from build123d import *

# Parameters (mm, degrees)
SKETCH1_R           = 11
SKETCH1_R_2         = 6.5
BOSS_EXTRUDE1_DEPTH = 2.75
SKETCH1_3_R         = 12.5
SKETCH1_3_R_2       = 11
SKETCH1_3_R_3       = 6.5
SKETCH1_3_R_4       = 5
BOSS_EXTRUDE2_DEPTH = 3
CHAMFER1_SIZE       = 0.3


with BuildPart() as part:
    # Sketch1 → Boss-Extrude1 (new, symmetric)
    with BuildSketch(Plane(origin=(0, 0, 0), x_dir=(1, 0, 0), z_dir=(0, 1, 0))):
        with Locations(Location((0, 0, 0), (0, 0, 270))):
            Circle(SKETCH1_R)
        with Locations(Location((0, 0, 0), (0, 0, 270))):
            Circle(SKETCH1_R_2, mode=Mode.SUBTRACT)
    extrude(amount=BOSS_EXTRUDE1_DEPTH, both=True)

    # Sketch1_3 → Boss-Extrude2 (add, symmetric)
    # profile 1 of 2: a face of its own
    with BuildSketch(Plane(origin=(0, 0, 0), x_dir=(1, 0, 0), z_dir=(0, 1, 0))):
        with Locations(Location((0, 0, 0), (0, 0, 270))):
            Circle(SKETCH1_3_R)
        with Locations(Location((0, 0, 0), (0, 0, 270))):
            Circle(SKETCH1_3_R_2, mode=Mode.SUBTRACT)
    # profile 2 of 2: a face of its own
    with BuildSketch(Plane(origin=(0, 0, 0), x_dir=(1, 0, 0), z_dir=(0, 1, 0))):
        with Locations(Location((0, 0, 0), (0, 0, 270))):
            Circle(SKETCH1_3_R_3)
        with Locations(Location((0, 0, 0), (0, 0, 270))):
            Circle(SKETCH1_3_R_4, mode=Mode.SUBTRACT)
    extrude(amount=BOSS_EXTRUDE2_DEPTH, both=True)

    # Chamfer1
    chamfer1_edges = [part.edges().sort_by_distance(p)[0] for p in [
        (0, 3, -12.5),
        (0, 3, -5),
        (0, -3, -5),
        (0, -3, -12.5),
    ]]
    chamfer(chamfer1_edges, length=CHAMFER1_SIZE)


solid = part.part
CAD build for the part. Positions are in the model's coordinates, mm. A direction names the side the tool comes from. Give positions to 0.01 mm unless a question says otherwise; leave off trailing zeros. Order: outer loops, then holes, each group sorted by start corner. A loop starts at its lowest first (then second) coordinate and runs counter-clockwise, first axis right, second up. Notation, with made-up numbers: (-13.5, 3.5) - (39.5, 3.5) arc R22 ccw to (39.5, 10.5) - close; hole circle Ø6 at (-20, -7). An arc over 180 degrees is marked (long way). Write each question's results on one line, items separated by ' | '.
1. Saw through at C-C on y = 1. List the corners of the cut face in (x, z), and give its area (3 significant figures).
Calculated:
outline: circle Ø25 at (0, 0); hole circle Ø10 at (0, 0) | area: 412 mm2
2. Pull direction X, two halves, no side cores. Call faces 1 (the face through (3.755, 0.038, 11.923)), 2 (the face through (-5, -2.75, 5)), 3 (the face through (11, -3, -2)): released by +X, released by -X, zero draft, split by the parting line, or undercut.
Calculated:
face 1: split by the parting line | face 2: undercut | face 3: zero draft
3. Probe L1, parallel to Z at x = 0.25, y = 1.2; L2, parallel to X at y = -1, z = 0; L3, parallel to Y at x = 7, z = -1.75. List the from-to ranges inside material, lowest first. Write a range as from..to.
Calculated:
L1: z = -12.5..-4.99, 4.99..12.5 | L2: x = -12.5..-5, 5..12.5 | L3: y = -2.75..2.75
4. Pin check, flat tips, straight feed: pin 1 (3 mm diameter, centred on y = -1.5, z = -2, fed in from -X); pin 2 (4 mm diameter, centred on x = 2.5, z = 8.5, fed in from +Y); pin 3 (1.5 mm diameter, centred on y = 0, z = 8, fed in from +X). Stop position of each tip, or through.
Calculated:
pin 1: stops at x = -12.49 | pin 2: stops at y = 2.75 | pin 3: stops at x = 10.18
5. 3-axis set-ups, long thin cutter, end or side, ignore diameter. For faces 4 (the face through (-5, 2.75, 5)), 5 (the face through (11, 3, -2)): which of +Z, -Z, +X, -X, +Y, -Y reach the whole face in a straight line?
Calculated:
face 4: +Y | face 5: +Z, -Z, +X, -X, +Y
